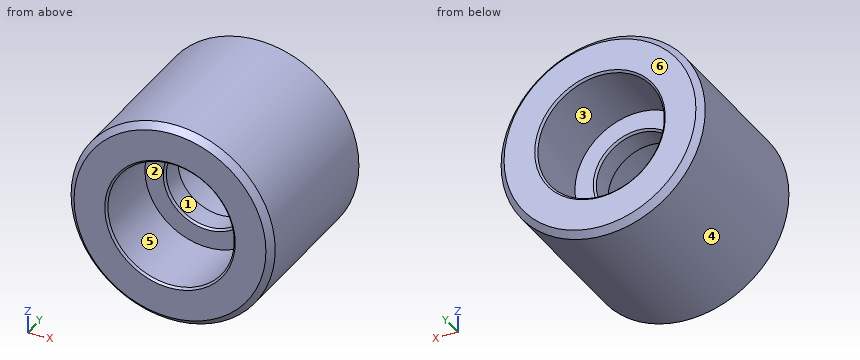
from build123d import *

# Parameters (mm, degrees)
F0_R        = 30.975
F0_R_2      = 21
F1_DEPTH    = 6.5
F0_R_3      = 50
F2_DEPTH    = 42.5
F2_FACE_R   = 50
F2_FACE_R_2 = 30.975
F3_DEPTH    = 42.5
F4_SIZE     = 3
F5_SIZE     = 1


with BuildPart() as f1:
    # F0 (on Front) → F1 (new body, symmetric)
    with BuildSketch(Plane.XZ):
        Circle(F0_R)
        Circle(F0_R_2, mode=Mode.SUBTRACT)
    extrude(amount=F1_DEPTH, both=True)

    # F0 (on Front) → F2 (join)
    with BuildSketch(Plane.XZ):
        Circle(F0_R_3)
        Circle(F0_R, mode=Mode.SUBTRACT)
    extrude(amount=F2_DEPTH)

    # F2_face (on face) → F3 (join)
    with BuildSketch(Plane(origin=(0, 0, 0), x_dir=(1, 0, 0), z_dir=(0, 1, 0))):
        Circle(F2_FACE_R)
        Circle(F2_FACE_R_2, mode=Mode.SUBTRACT)
    extrude(amount=F3_DEPTH)

    # F4
    f4_edges = [f1.edges().sort_by_distance(p)[0] for p in [
        (-50, 42.5, 0),
        (-50, -42.5, 0),
    ]]
    chamfer(f4_edges, length=F4_SIZE)

    # F5
    f5_edges = [f1.edges().sort_by_distance(p)[0] for p in [
        (-30.975, 42.5, 0),
        (-21, 6.5, 0),
        (-21, -6.5, 0),
        (-30.975, -42.5, 0),
    ]]
    chamfer(f5_edges, length=F5_SIZE)


solid = f1.part
Geometry: final body of the model. Coordinates: model frame, mm. Face numbers are marked on the shaded views. A direction names the side the tool comes from. Give positions to 0.01 mm unless a question says otherwise; leave off trailing zeros. Write each loop counter-clockwise with the first axis right and the second up, starting at its lowest first coordinate (ties: lowest second). Pieces come first, ordered by that corner, then holes.
(1) Access query for the marked faces 1, 2 and 3. Directions: +Z, -Z, +X, -X, +Y, -Y. A direction counts if a zero-diameter tool reaches every point of the face in a straight line with its end or side. Return the directions, or none.
(2) Cut plane D-D, the plane y = 3. Return loops of the section in (x, z).
(3) Ray query, line 1 (X direction, y = 29.5, z = 0) (3 decimals); line 2 (Z direction, x = 0, y = 2). Return the intervals inside material, ascending.
(4) First-contact query: P1, Ø4, axis at x = -34.5, y = 24.5, coming from the +Z side; P2, Ø1.5, axis at x = -21, z = 9, coming from the -Y side; P3, Ø1.5, axis at y = 5.5, z = 22, coming from the -X side. Flat tips, straight axial feed; report the tip coordinate or a pass-through.
(5) Mould query, pull axis X, two halves, no side actions, for the marked faces 4, 5 and 6. Classes: released by +X, released by -X, zero draft, split by the parting line, or undercut.
(6) Cut plane C-C, the plane y = 31.5. Return loops of the section in (x, z) (3 decimals).
(7) Cut plane A-A, the plane z = 0. Return loops of the section in (x, y) (3 decimals).
(8) Cut plane B-B, the plane x = 0. Return loops of the section in (y, z) (3 decimals).
Values follow:
1. face 1: +Y, -Y
1. face 2: -Y
1. face 3: +Y
2. outline: circle Ø100 at (0, 0); hole circle Ø42 at (0, 0)
3. line 1: x = -50 to -30.975, 30.975 to 50
3. line 2: z = -50 to -21, 21 to 50
4. P1: stops at z = 38
4. P2: stops at y = -6.5
4. P3: stops at x = -45.26
5. face 4: split by the parting line
5. face 5: undercut
5. face 6: zero draft
6. outline: circle Ø100 at (0, 0); hole circle Ø61.95 at (0, 0)
7. outline: (-50, -39.5) - (-47, -42.5) - (-31.975, -42.5) - (-30.975, -41.5) - (-30.975, -6.5) - (-22, -6.5) - (-21, -5.5) - (-21, 5.5) - (-22, 6.5) - (-30.975, 6.5) - (-30.975, 41.5) - (-31.975, 42.5) - (-47, 42.5) - (-50, 39.5) - close; (21, -5.5) - (22, -6.5) - (30.975, -6.5) - (30.975, -41.5) - (31.975, -42.5) - (47, -42.5) - (50, -39.5) - (50, 39.5) - (47, 42.5) - (31.975, 42.5) - (30.975, 41.5) - (30.975, 6.5) - (22, 6.5) - (21, 5.5) - close
8. outline: (-42.5, -47) - (-39.5, -50) - (39.5, -50) - (42.5, -47) - (42.5, -31.975) - (41.5, -30.975) - (6.5, -30.975) - (6.5, -22) - (5.5, -21) - (-5.5, -21) - (-6.5, -22) - (-6.5, -30.975) - (-41.5, -30.975) - (-42.5, -31.975) - close; (-42.5, 31.975) - (-41.5, 30.975) - (-6.5, 30.975) - (-6.5, 22) - (-5.5, 21) - (5.5, 21) - (6.5, 22) - (6.5, 30.975) - (41.5, 30.975) - (42.5, 31.975) - (42.5, 47) - (39.5, 50) - (-39.5, 50) - (-42.5, 47) - close
